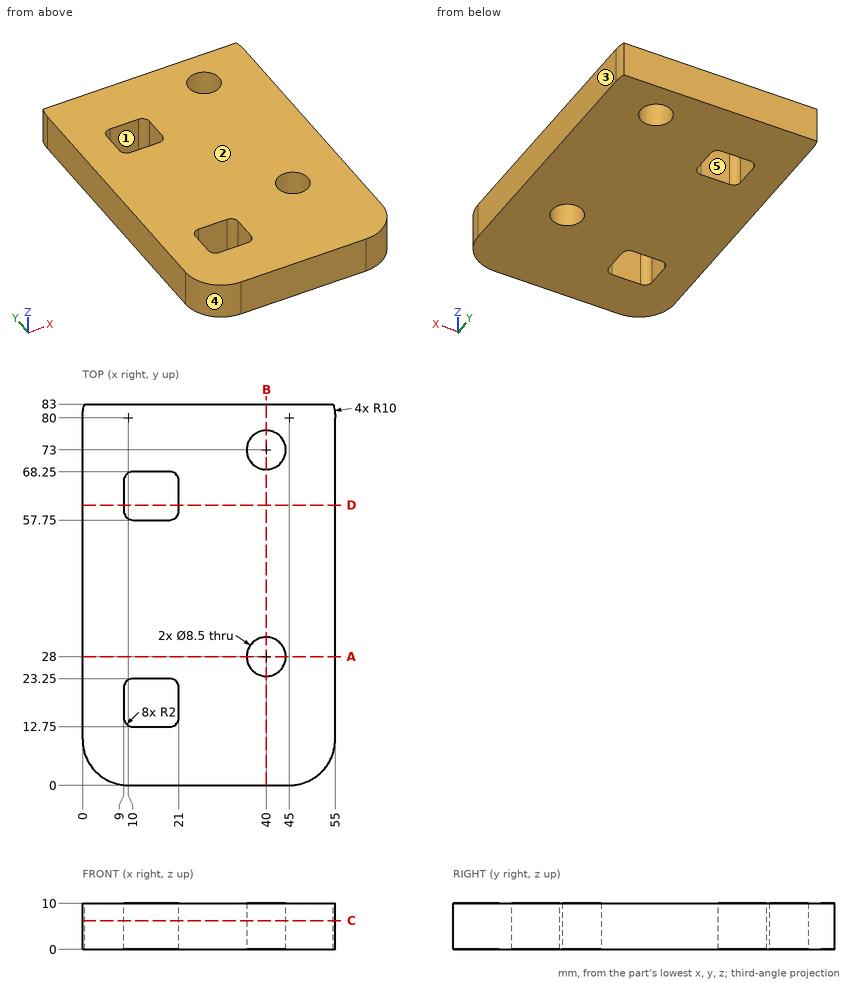
Answer from the drawing. Dimensions are ordinates in mm from the lowest x, y and z of the part. A direction names the side the tool comes from. Give positions to 0.01 mm unless a question says otherwise; leave off trailing zeros. Loops run counter-clockwise (first coordinate to the right, second up) from the corner with the lowest first, then second, coordinate; pieces in that order, holes last. Notation, with made-up numbers: (-31, 59.25) - (16, 59.25) arc R18 ccw to (16, 78.25) - close; hole circle Ø6 at (70, 14). An arc over 180 degrees is marked (long way). Answer as CSV lines item,"result". Start each with the question number.
Item 1: A cutting plane is placed at C-C on z = 6.25. Determine the outline of the cut face in (x, y), then the cut area to 3 significant figures.
Item 2: A cutting plane is placed at B-B on x = 40. Determine the outline of the cut face in (y, z).
Item 3: The mould has two halves that part along X. Classify the marked faces 3, 4 and 5: +X half, -X half, draft (parallel to the pull), parting line (faces both ways), or undercut.
Item 4: Each of these flat-tipped pins is pushed along its axis until it touches: pin 1 (6 mm diameter, centred on x = 6.5, y = 40, fed in from -Z); pin 2 (7.5 mm diameter, centred on x = 40, y = 28, fed in from -Z). Where does it stop, or does it pass through?
Item 5: Find the intervals of material crossed by line 1 (Y direction, x = 40, z = 6.25); line 2 (Y direction, x = 16, z = 7.5); line 3 (X direction, y = 69.5, z = 1), in increasing order. Write a range as from..to.
Item 6: For the marked faces 1 and 2, determine the directions among +Z, -Z, +X, -X, +Y, -Y from which every point of the face is accessible in a straight line to the end or side of a thin tool.
Item 7: A cutting plane is placed at D-D on y = 61. Determine the outline of the cut face in (x, z).
Item 8: A cutting plane is placed at A-A on y = 28. Determine the outline of the cut face in (x, z).
Found:
1,outline,"(0, 10) arc R10 ccw to (10, 0) - (45, 0) arc R10 ccw to (55, 10) - (55, 80) arc R10 ccw to (54.54, 83) - (0.46, 83) arc R10 ccw to (0, 80) - close; hole (9, 14.75) arc R2 ccw to (11, 12.75) - (19, 12.75) arc R2 ccw to (21, 14.75) - (21, 21.25) arc R2 ccw to (19, 23.25) - (11, 23.25) arc R2 ccw to (9, 21.25) - close; hole (9, 59.75) arc R2 ccw to (11, 57.75) - (19, 57.75) arc R2 ccw to (21, 59.75) - (21, 66.25) arc R2 ccw to (19, 68.25) - (11, 68.25) arc R2 ccw to (9, 66.25) - close; hole circle Ø8.5 at (40, 28); hole circle Ø8.5 at (40, 73)"
1,area,"4,160 mm^2"
2,outline,"(0, 0) - (23.75, 0) - (23.75, 10) - (0, 10) - close; (32.25, 0) - (68.75, 0) - (68.75, 10) - (32.25, 10) - close; (77.25, 0) - (83, 0) - (83, 10) - (77.25, 10) - close"
3,face 3,"+X half"
3,face 4,"-X half"
3,face 5,"undercut"
4,pin 1,"stops at z = 0"
4,pin 2,"passes through"
5,line 1,"y = 0..23.75, 32.25..68.75, 77.25..83"
5,line 2,"y = 0..12.75, 23.25..57.75, 68.25..83"
5,line 3,"x = 0..37.59, 42.41..55"
6,face 1,"+Z, -Z"
6,face 2,"+Z, +X, -X, +Y, -Y"
7,outline,"(0, 0) - (9, 0) - (9, 10) - (0, 10) - close; (21, 0) - (55, 0) - (55, 10) - (21, 10) - close"
8,outline,"(0, 0) - (35.75, 0) - (35.75, 10) - (0, 10) - close; (44.25, 0) - (55, 0) - (55, 10) - (44.25, 10) - close"
